Read the model definition and answer for the solid it produces. Units are mm, in the model's axes. Face numbers are marked on the shaded views. Give positions to 0.01 mm unless a question says otherwise; leave off trailing zeros. Loops run counter-clockwise (first coordinate to the right, second up) from the corner with the lowest first, then second, coordinate; pieces in that order, holes last. Notation, with made-up numbers: (33, 88) - (37, 88) arc R15 cw to (37, 110) - close; hole circle Ø2 at (-11.5, 57). An arc over 180 degrees is marked (long way). Use a Markdown table: item, result. Add a question column.
Item 1: For a pull along X with two mould halves and no side action, classify the marked faces 1 and 2 as +X half, -X half, draft (parallel to the pull), parting line (faces both ways), or undercut.
Item 2: A cutting plane is placed at B-B (x = 92). Determine the outline of the cut face in (y, z), plus the area to 3 significant figures.
Item 3: Each of these flat-tipped pins is pushed along its axis until it touches: P1, Ø1.5, axis at y = 9.5, z = 2, coming from the -X side; P2, Ø1.5, axis at x = 86.5, y = 0, coming from the +Z side; P3, Ø0.8, axis at y = 7, z = 1.5, coming from the +X side. Where does it stop, or does it pass through?
Item 4: A cutting plane is placed at A-A (z = 1.75). Give the number of separate pieces and of enclosed holes in the cut face, plus the area to 3 significant figures.
Item 5: A cutting plane is placed at C-C (y = -2). Determine the outline of the cut face in (x, z), plus the area to 3 significant figures.
Item 6: Consider probe 1 along X at (y, z) = (2, 2.2); probe 2 along Z at (x, y) = (30, 14.5); probe 3 along Y at (x, z) = (48, 1.6). Determine where each line is inside the solid, lowest interval first. Write a range as [from, to].
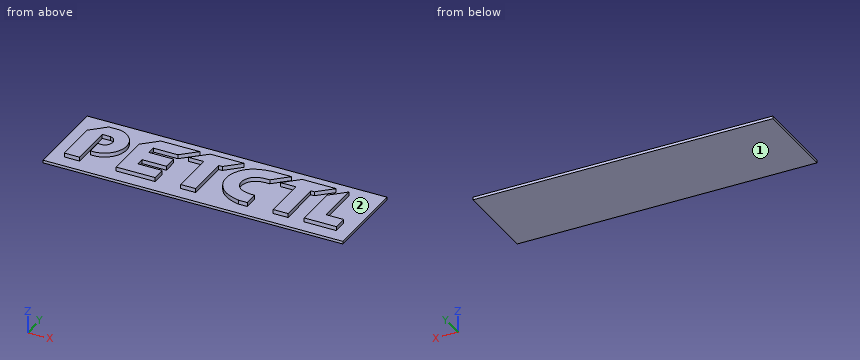
from build123d import *

# Parameters (mm, degrees)
SKETCH_W     = 110.04
SKETCH_H     = 31.13
PAD_DEPTH    = 1
PAD001_DEPTH = 1.5


with BuildPart() as part:
    # Sketch → Pad (new body)
    with BuildSketch(Plane.XY):
        with Locations((50.02, 10.565)):
            Rectangle(SKETCH_W, SKETCH_H)
    extrude(amount=PAD_DEPTH)

    # Sketch001 → Pad001 (join)
    with BuildSketch(Plane.XY.offset(1)):
        with BuildLine():
            Line((9.050295, 10.321073), (7.066321, 10.321073))
            Line((7.066321, 10.321073), (7.066321, 5.163982))
            ThreePointArc((7.066321, 5.163982), (16.188383, 12.014691), (9.330203, 21.131137))
            Line((9.330203, 21.131137), (5.608163, 21.131137))
            Line((5.608163, 21.131137), (0.205283, 16.081137))
            Line((0.205283, 16.081137), (0.205283, 0))
            Line((0.205283, 0), (5.809592, 0))
            Line((5.809592, 0), (5.809592, 16.015693))
            Line((5.809592, 16.015693), (8.888276, 16.015693))
            ThreePointArc((8.888276, 16.015693), (11.152955, 13.230511), (9.050295, 10.321073))
        make_face()
        with BuildLine():
            add(Edge.make_bspline(
                [(67.303898, 15.965996), (62.098309, 16.191984), (58.974827, 11.8324), (60.112492, 7.371485), (63.086761, 5.170527), (67.363525, 5.130735)],
                knots=[0, 0, 0, 0, 0.333333, 0.666667, 1, 1, 1, 1], degree=3))
            Line((67.363525, 5.130735), (67.363525, 0))
            Line((67.363525, 0), (64.118454, 0))
            add(Edge.make_bspline(
                [(65.6586, 21.015996), (59.749424, 20.528551), (54.754429, 16.165611), (53.644032, 9.523063), (55.59515, 4.427975), (59.316757, 1.105113), (64.118454, 0)],
                knots=[0, 0, 0, 0, 0.25, 0.5, 0.75, 1, 1, 1, 1], degree=3))
            Line((65.6586, 21.015996), (72.706779, 21.015996))
            Line((72.706779, 21.015996), (67.303898, 15.965996))
        make_face()
        Polygon((38.950399, 21.12416), (24.620772, 21.12416), (19.217891, 16.07416), (19.217891, 0), (33.507112, 0), (33.507112, 5.05), (24.537624, 5.05), (24.537624, 7.978263), (33.507112, 7.978263), (33.507112, 13.028263), (24.537624, 13.028263), (24.537624, 16.07416), (33.547518, 16.07416), align=None)
        Polygon((42.687428, 21.282697), (37.284547, 16.232697), (42.935597, 16.232697), (42.935597, 0), (48.416265, 0), (48.416265, 16.232697), (49.751421, 16.232697), (55.154302, 21.282697), align=None)
        Polygon((76.574252, 21.071087), (71.171371, 16.021087), (76.822421, 16.021087), (76.822421, 0), (82.303089, 0), (82.303089, 16.021087), (83.638245, 16.021087), (89.041126, 21.071087), align=None)
        Polygon((88.247359, 16.026386), (93.65024, 21.076386), (93.682304, 5.090163), (100.043274, 5.090163), (100.043274, 0), (88.247359, 0), align=None)
    extrude(amount=PAD001_DEPTH)


solid = part.part
Geometry says:
| question | item | result |
|---|---|---|
| 1 | face 1 | draft |
| 1 | face 2 | undercut |
| 2 | outline | (-5, 0) - (26.13, 0) - (26.13, 1) - (19.53, 1) - (19.53, 2.5) - (0, 2.5) - (0, 1) - (-5, 1) - close |
| 2 | area | 60.4 mm² |
| 3 | P1 | x = 0.21 |
| 3 | P2 | z = 1 |
| 3 | P3 | x = 93.68 |
| 4 | separate pieces | 6 |
| 4 | enclosed holes | 0 |
| 4 | area | 1,070 mm² |
| 5 | outline | (-5, 0) - (105.04, 0) - (105.04, 1) - (-5, 1) - close |
| 5 | area | 110 mm² |
| 6 | probe 1 | [0.21, 5.81], [19.22, 33.51], [42.94, 48.42], [58.84, 67.36], [76.82, 82.3], [88.25, 100.04] |
| 6 | probe 2 | [0, 1] |
| 6 | probe 3 | [0, 21.28] |
